CAD build for the part. Positions are in the model's coordinates, mm. Face numbers are marked on the shaded views. A direction names the side the tool comes from. Round coordinates to 2 decimals unless told otherwise and drop trailing zeros. Order: outer loops, then holes, each group sorted by start corner. A loop starts at its lowest first (then second) coordinate and runs counter-clockwise, first axis right, second up. Notation, with made-up numbers: (24, 40.25) - (34, 40.25) arc R9 cw to (34, 47.25) - close; hole circle Ø2 at (0.25, 57). An arc over 180 degrees is marked (long way). Write item = value, one per line.
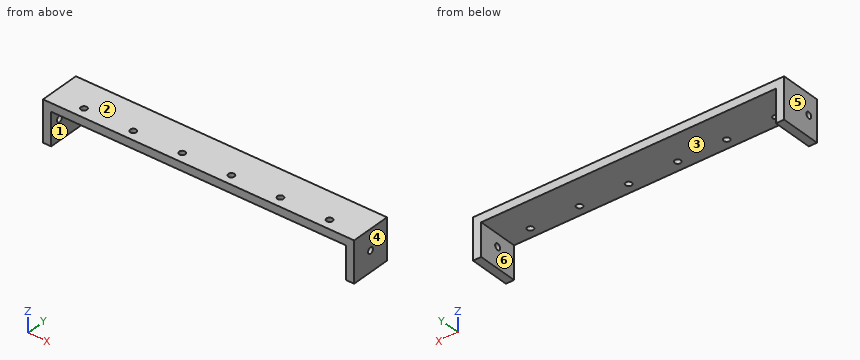
from build123d import *

# Parameters (mm, degrees)
SKETCH1_W           = 72
SKETCH1_H           = 10
BOSS_EXTRUDE1_DEPTH = 2
SKETCH3_R           = 0.75
CUT_EXTRUDE2_DEPTH  = 2
SKETCH4_W           = 10
SKETCH4_H           = 10
BOSS_EXTRUDE2_DEPTH = 2
SKETCH5_R           = 0.75
CUT_EXTRUDE4_DEPTH  = 2
SKETCH6_W           = 10
SKETCH6_H           = 10
BOSS_EXTRUDE3_DEPTH = 2
SKETCH7_R           = 0.75
CUT_EXTRUDE5_DEPTH  = 2


with BuildPart() as part:
    # Sketch1 → Boss-Extrude1 (new body)
    with BuildSketch(Plane.XY):
        with Locations((36, 5)):
            Rectangle(SKETCH1_W, SKETCH1_H)
    extrude(amount=BOSS_EXTRUDE1_DEPTH)

    # Sketch3 → Cut-Extrude2 (cut)
    with BuildSketch(Plane.XY):
        with Locations((42, 2.5)):
            Circle(SKETCH3_R)
        with Locations((54, 2.5)):
            Circle(SKETCH3_R)
        with Locations((66, 2.5)):
            Circle(SKETCH3_R)
        with Locations((30, 2.5)):
            Circle(SKETCH3_R)
        with Locations((18.06024044, 2.463599586)):
            Circle(SKETCH3_R)
        with Locations((6, 2.5)):
            Circle(SKETCH3_R)
    extrude(amount=CUT_EXTRUDE2_DEPTH, mode=Mode.SUBTRACT)

    # Sketch4 → Boss-Extrude2 (add)
    with BuildSketch(Plane(origin=(72, 0, 0), x_dir=(0, 0, -1), z_dir=(1, 0, 0))):
        with Locations((3, 5)):
            Rectangle(SKETCH4_W, SKETCH4_H)
    extrude(amount=BOSS_EXTRUDE2_DEPTH)

    # Sketch5 → Cut-Extrude4 (cut)
    with BuildSketch(Plane(origin=(72, 0, 0), x_dir=(0, 0, -1), z_dir=(1, 0, 0))):
        with Locations((3, 5)):
            Circle(SKETCH5_R)
    extrude(amount=CUT_EXTRUDE4_DEPTH, mode=Mode.SUBTRACT)

    # Sketch6 → Boss-Extrude3 (add)
    with BuildSketch(Plane.ZY):
        with Locations((-3, 5)):
            Rectangle(SKETCH6_W, SKETCH6_H)
    extrude(amount=BOSS_EXTRUDE3_DEPTH)

    # Sketch7 → Cut-Extrude5 (cut)
    with BuildSketch(Plane.ZY):
        with Locations((-3, 2.5)):
            Circle(SKETCH7_R)
    extrude(amount=CUT_EXTRUDE5_DEPTH, mode=Mode.SUBTRACT)


solid = part.part
(1) Probe line 1 along X through (y, z) = (3.5, -1.5); line 2 along Y through (x, z) = (-0.7, -3); line 3 along Z through (x, y) = (19.5, 2.75). List the from-to ranges inside material, lowest first.
Solved:
line_1 = -2 to 0, 72 to 74
line_2 = 0 to 1.75, 3.25 to 10
line_3 = 0 to 2
(2) Pull direction X, two halves, no side cores. Call the marked faces 1, 2, 3 and 4: released by +X, released by -X, zero draft, split by the parting line, or undercut.
Solved:
face_1 = undercut
face_2 = zero draft
face_3 = undercut
face_4 = released by +X
(3) Drop flat-ended pins along their axis: pin 1 (0.9 mm diameter, centred on x = 6, y = 2.5, fed in from -Z); pin 2 (2 mm diameter, centred on x = 42, y = 2.5, fed in from -Z); pin 3 (1.4 mm diameter, centred on y = 2.5, z = -3, fed in from -X). Give the stop position or say it passes through.
Solved:
pin_1 = through
pin_2 = 0
pin_3 = 72
(4) Band-saw the part on D-D on y = 1. List the corners of the cut face in (x, z), plus the area to 3 significant figures.
Solved:
outline = (-2, -8) - (0, -8) - (0, 0) - (72, 0) - (72, -8) - (74, -8) - (74, 2) - (-2, 2) - close
area = 184 mm²
(5) Band-saw the part on C-C on y = 5. List the corners of the cut face in (x, z), plus the area to 3 significant figures.
Solved:
outline = (-2, -8) - (0, -8) - (0, 0) - (72, 0) - (72, -2.25) - (74, -2.25) - (74, 2) - (-2, 2) - close; (72, -8) - (74, -8) - (74, -3.75) - (72, -3.75) - close
area = 181 mm²
(6) Tool access for the marked faces 5 and 6: list every direction of +Z, -Z, +X, -X, +Y, -Y with a clear straight run to the whole face (end or side of a thin tool).
Solved:
face_5 = +Z, -Z, -X, +Y, -Y
face_6 = -Z, +Y, -Y
(7) Band-saw the part on A-A on z = -0.75. List the corners of the cut face in (x, y), plus the area to 3 significant figures.
Solved:
outline = (-2, 0) - (0, 0) - (0, 10) - (-2, 10) - close; (72, 0) - (74, 0) - (74, 10) - (72, 10) - close
area = 40.0 mm²
(8) Band-saw the part on B-B on x = 30. List the corners of the cut face in (y, z), plus the area to 3 significant figures.
Solved:
outline = (0, 0) - (1.75, 0) - (1.75, 2) - (0, 2) - close; (3.25, 0) - (10, 0) - (10, 2) - (3.25, 2) - close
area = 17.0 mm²
